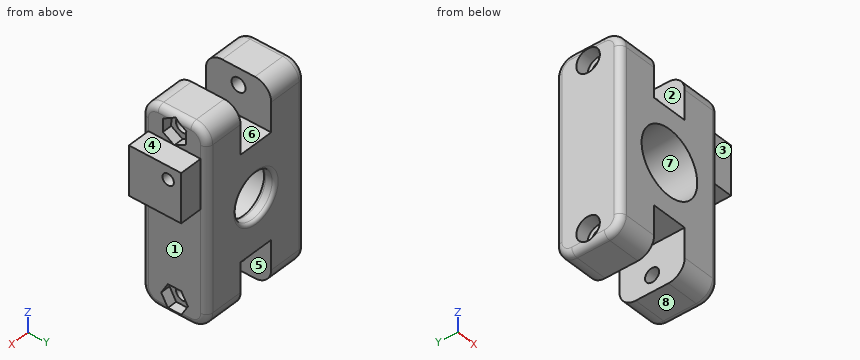
from build123d import *

# Parameters (mm, degrees)
SKETCH1_W           = 35
SKETCH1_H           = 60
BOSS_EXTRUDE1_DEPTH = 20
SKETCH2_R           = 10
CUT_EXTRUDE1_DEPTH  = 16
SKETCH4_R           = 7
CUT_EXTRUDE2_DEPTH  = 42.997755111
FILLET1_R           = 2
SKETCH5_W           = 11
SKETCH5_H           = 14
CUT_EXTRUDE3_DEPTH  = 44.678500826
SKETCH6_R           = 2.15
CUT_EXTRUDE4_DEPTH  = 53.234749007
FILLET3_R           = 5
FILLET4_R           = 5
FILLET7_R           = 1
SKETCH9_W           = 15
SKETCH9_H           = 16
BOSS_EXTRUDE3_DEPTH = 7
SKETCH10_R          = 1.75
CUT_EXTRUDE6_DEPTH  = 5
SKETCH12_R          = 3.6
CUT_EXTRUDE7_DEPTH  = 4
CUT_EXTRUDE8_DEPTH  = 3


with BuildPart() as part:
    # Sketch1 → Boss-Extrude1 (new body)
    with BuildSketch(Plane(origin=(0, 0, 0), x_dir=(1, 0, 0), z_dir=(0, 1, 0))):
        with Locations((-2.608267717, 3.218503937)):
            Rectangle(SKETCH1_W, SKETCH1_H)
    extrude(amount=BOSS_EXTRUDE1_DEPTH)

    # Sketch2 → Cut-Extrude1 (cut)
    with BuildSketch(Plane.XZ):
        with Locations(Location((-2.608267717, -3.218503937, 0), (0, 0, 270))):
            Circle(SKETCH2_R)
    extrude(amount=-CUT_EXTRUDE1_DEPTH, mode=Mode.SUBTRACT)

    # Sketch4 → Cut-Extrude2 (cut, through all)
    with BuildSketch(Plane.XZ.offset(-16)):
        with Locations(Location((-2.608267717, -3.218503937, 0), (0, 0, 270))):
            Circle(SKETCH4_R)
    extrude(amount=-CUT_EXTRUDE2_DEPTH, mode=Mode.SUBTRACT)

    # Fillet1
    fillet1_edges = [part.edges().sort_by_distance(p)[0] for p in [
        (-20.108267717, 20, -3.218503937),
        (14.891732283, 20, -3.218503937),
        (-20.108267717, 0, -3.218503937),
        (14.891732283, 0, -3.218503937),
        (14.891732283, 10, 26.781496063),
        (-20.108267717, 10, 26.781496063),
        (-20.108267717, 10, -33.218503937),
        (14.891732283, 10, -33.218503937),
    ]]
    fillet(fillet1_edges, radius=FILLET1_R)

    # Sketch5 → Cut-Extrude3 (cut, through all)
    with BuildSketch(Plane.XZ):
        with Locations((-2.608267717, 19.781496063)):
            Rectangle(SKETCH5_W, SKETCH5_H)
        with Locations((-2.608267717, -26.218503937)):
            Rectangle(SKETCH5_W, SKETCH5_H)
    extrude(amount=-CUT_EXTRUDE3_DEPTH, mode=Mode.SUBTRACT)

    # Sketch6 → Cut-Extrude4 (cut, through all)
    with BuildSketch(Plane.ZY.offset(20.108267717)):
        with Locations((-28.218503937, 10)):
            Circle(SKETCH6_R)
        with Locations((21.781496063, 10)):
            Circle(SKETCH6_R)
    extrude(amount=-CUT_EXTRUDE4_DEPTH, mode=Mode.SUBTRACT)

    # Fillet3
    # the kernel refuses this fillet: 5 mm, written as the material it takes off along each edge
    with BuildSketch(Plane(origin=(-20.108267717, 15, 21.781496063), x_dir=(0, 0, 1), z_dir=(0, -1, 0))) as fillet3_piece_1:
        with BuildLine():
            CenterArc((3, -2), 2, 0, 90)
            Line((5, -2), (5, 0))
            Line((5, 0), (3, 0))
        make_face()
    revolve(axis=Axis((-20.108267717, 15, 21.781496063), (-1, 0, 0)), revolution_arc=90, mode=Mode.SUBTRACT)
    with BuildSketch(Plane(origin=(-20.108267717, 5, 21.781496063), x_dir=(0, -1, 0), z_dir=(0, 0, -1))) as fillet3_piece_2:
        with BuildLine():
            CenterArc((3, -2), 2, 0, 90)
            Line((5, -2), (5, 0))
            Line((5, 0), (3, 0))
        make_face()
    revolve(axis=Axis((-20.108267717, 5, 21.781496063), (-1, 0, 0)), revolution_arc=90, mode=Mode.SUBTRACT)
    with BuildSketch(Plane(origin=(14.891732283, 15, 21.781496063), x_dir=(0, 1, 0), z_dir=(0, 0, -1))) as fillet3_piece_3:
        with BuildLine():
            CenterArc((3, -2), 2, 0, 90)
            Line((5, -2), (5, 0))
            Line((5, 0), (3, 0))
        make_face()
    revolve(axis=Axis((14.891732283, 15, 21.781496063), (1, 0, 0)), revolution_arc=90, mode=Mode.SUBTRACT)
    with BuildSketch(Plane(origin=(14.891732283, 5, 21.781496063), x_dir=(0, 0, 1), z_dir=(0, 1, 0))) as fillet3_piece_4:
        with BuildLine():
            CenterArc((3, -2), 2, 0, 90)
            Line((5, -2), (5, 0))
            Line((5, 0), (3, 0))
        make_face()
    revolve(axis=Axis((14.891732283, 5, 21.781496063), (1, 0, 0)), revolution_arc=90, mode=Mode.SUBTRACT)
    with BuildSketch(Plane(origin=(4.391732283, 20, 26.781496063), x_dir=(0, 0, -1), z_dir=(-1, 0, 0)), Plane(origin=(14.891732283, 0, 26.781496063), x_dir=(0, 1, 0), z_dir=(-1, 0, 0))) as fillet3_piece_5:
        with BuildLine():
            CenterArc((FILLET3_R, FILLET3_R), FILLET3_R, 180, 90)
            Line((0, FILLET3_R), (0, 0))
            Line((0, 0), (FILLET3_R, 0))
        make_face()
    extrude(amount=24.5, mode=Mode.SUBTRACT)
    with BuildSketch(Plane(origin=(4.391732283, 0, 26.781496063), x_dir=(0, 0, -1), z_dir=(-1, 0, 0)), Plane(origin=(14.891732283, 20, 26.781496063), x_dir=(0, -1, 0), z_dir=(-1, 0, 0))) as fillet3_piece_6:
        with BuildLine():
            CenterArc((FILLET3_R, -FILLET3_R), FILLET3_R, 90, 90)
            Line((0, -FILLET3_R), (0, 0))
            Line((0, 0), (FILLET3_R, 0))
        make_face()
    extrude(amount=24.5, mode=Mode.SUBTRACT)

    # Fillet4
    # the kernel refuses this fillet: 5 mm, written as the material it takes off along each edge
    with BuildSketch(Plane(origin=(-20.108267717, 15, -28.218503937), x_dir=(0, 1, 0), z_dir=(0, 0, 1))) as fillet4_piece_1:
        with BuildLine():
            CenterArc((3, -2), 2, 0, 90)
            Line((5, -2), (5, 0))
            Line((5, 0), (3, 0))
        make_face()
    revolve(axis=Axis((-20.108267717, 15, -28.218503937), (-1, 0, 0)), revolution_arc=90, mode=Mode.SUBTRACT)
    with BuildSketch(Plane(origin=(-20.108267717, 5, -28.218503937), x_dir=(0, 0, -1), z_dir=(0, 1, 0))) as fillet4_piece_2:
        with BuildLine():
            CenterArc((3, -2), 2, 0, 90)
            Line((5, -2), (5, 0))
            Line((5, 0), (3, 0))
        make_face()
    revolve(axis=Axis((-20.108267717, 5, -28.218503937), (-1, 0, 0)), revolution_arc=90, mode=Mode.SUBTRACT)
    with BuildSketch(Plane(origin=(14.891732283, 15, -28.218503937), x_dir=(0, 0, -1), z_dir=(0, -1, 0))) as fillet4_piece_3:
        with BuildLine():
            CenterArc((3, -2), 2, 0, 90)
            Line((5, -2), (5, 0))
            Line((5, 0), (3, 0))
        make_face()
    revolve(axis=Axis((14.891732283, 15, -28.218503937), (1, 0, 0)), revolution_arc=90, mode=Mode.SUBTRACT)
    with BuildSketch(Plane(origin=(14.891732283, 5, -28.218503937), x_dir=(0, -1, 0), z_dir=(0, 0, 1))) as fillet4_piece_4:
        with BuildLine():
            CenterArc((3, -2), 2, 0, 90)
            Line((5, -2), (5, 0))
            Line((5, 0), (3, 0))
        make_face()
    revolve(axis=Axis((14.891732283, 5, -28.218503937), (1, 0, 0)), revolution_arc=90, mode=Mode.SUBTRACT)
    with BuildSketch(Plane(origin=(-9.608267717, 0, -33.218503937), x_dir=(0, 1, 0), z_dir=(1, 0, 0)), Plane(origin=(-20.108267717, 0, -33.218503937), x_dir=(0, 1, 0), z_dir=(1, 0, 0))) as fillet4_piece_5:
        with BuildLine():
            CenterArc((FILLET4_R, FILLET4_R), FILLET4_R, 180, 90)
            Line((0, FILLET4_R), (0, 0))
            Line((0, 0), (FILLET4_R, 0))
        make_face()
    extrude(amount=24.5, mode=Mode.SUBTRACT)
    with BuildSketch(Plane(origin=(-9.608267717, 20, -33.218503937), x_dir=(0, -1, 0), z_dir=(1, 0, 0)), Plane(origin=(-20.108267717, 20, -33.218503937), x_dir=(0, -1, 0), z_dir=(1, 0, 0))) as fillet4_piece_6:
        with BuildLine():
            CenterArc((FILLET4_R, -FILLET4_R), FILLET4_R, 90, 90)
            Line((0, -FILLET4_R), (0, 0))
            Line((0, 0), (FILLET4_R, 0))
        make_face()
    extrude(amount=24.5, mode=Mode.SUBTRACT)

    # Fillet7
    fillet7_edges = [part.edges().sort_by_distance(p)[0] for p in [
        (-2.608267717, 20, 3.781496063),
        (-2.608267717, 16, 3.781496063),
    ]]
    fillet(fillet7_edges, radius=FILLET7_R)

    # Sketch9 → Boss-Extrude3 (add)
    with BuildSketch(Plane(origin=(14.891732283, 0, 0), x_dir=(0, 0, -1), z_dir=(1, 0, 0))):
        with Locations((-10.281496063, 10)):
            Rectangle(SKETCH9_W, SKETCH9_H)
    extrude(amount=BOSS_EXTRUDE3_DEPTH)

    # Sketch10 → Cut-Extrude6 (cut)
    with BuildSketch(Plane(origin=(21.891732283, 0, 0), x_dir=(0, 0, -1), z_dir=(1, 0, 0))):
        with Locations((-13.781496063, 14)):
            Circle(SKETCH10_R)
    extrude(amount=-CUT_EXTRUDE6_DEPTH, mode=Mode.SUBTRACT)

    # Sketch12 → Cut-Extrude7 (cut)
    with BuildSketch(Plane.ZY.offset(20.108267717)):
        with Locations((-28.218503937, 10)):
            Circle(SKETCH12_R)
        with Locations((21.781496063, 10)):
            Circle(SKETCH12_R)
    extrude(amount=-CUT_EXTRUDE7_DEPTH, mode=Mode.SUBTRACT)

    # Sketch13 → Cut-Extrude8 (cut)
    with BuildSketch(Plane(origin=(14.891732283, 0, 0), x_dir=(0, 0, -1), z_dir=(1, 0, 0))):
        Polygon((-19.793991712, 6.414869628), (-17.682929909, 9.928664072), (-19.67043426, 13.513794445), (-23.769000414, 13.585130372), (-25.880062217, 10.071335928), (-23.892557866, 6.486205555), align=None)
        Polygon((28.218503937, 5.900813089), (31.768503937, 7.950406544), (31.768503937, 12.049593456), (28.218503937, 14.099186911), (24.668503937, 12.049593456), (24.668503937, 7.950406544), align=None)
    extrude(amount=-CUT_EXTRUDE8_DEPTH, mode=Mode.SUBTRACT)


solid = part.part
Input: part model. Units: mm. Frame: model coordinates. Face numbers are marked on the shaded views. A direction names the side the tool comes from. Coordinates: 2 decimals unless noted, no trailing zeros. Loops run counter-clockwise (first coordinate to the right, second up) from the corner with the lowest first, then second, coordinate; pieces in that order, holes last. Notation, with made-up numbers: (-25.75, 0) -> (-0.75, 0) arc R7 ccw to (-0.75, 6) -> close; hole circle Ø3 at (66.5, -28.5). An arc over 180 degrees is marked (long way). One line per item, written item: value.
(1) Set-up query: the marked faces 1, 2, 3, 4 and 5. Return all of +Z, -Z, +X, -X, +Y, -Y with unobstructed straight access to the full face (end or side cutting, diameter ignored); none if empty.
Answer below:
face 1: -Z, +X, +Y, -Y
face 2: +Z, +Y, -Y
face 3: +Z, -Z, +X, -Y
face 4: +Z, +X, +Y, -Y
face 5: -Z, +Y, -Y
(2) Cut plane C-C (z = 10.5). Output: boundary loops of the cut face in (x, y), then the cut area to 3 significant figures.
Answer below:
outline: (-20.11, 2) arc R2 ccw to (-18.11, 0) -> (12.89, 0) arc R2 ccw to (14.89, 2) -> (21.89, 2) -> (21.89, 18) -> (14.89, 18) arc R2 ccw to (12.89, 20) -> (-18.11, 20) arc R2 ccw to (-20.11, 18) -> close
area: 809 mm2
(3) Draft query along Z for the marked faces 6, 7 and 8. Return one class per face: pulls with the +Z half, pulls with the -Z half, needs draft (parallel to the pull), parting line crosses it, or undercut.
Answer below:
face 6: pulls with the +Z half
face 7: undercut
face 8: pulls with the -Z half
(4) Ray query, line 1 along X through (y, z) = (14.5, -30); line 2 along X through (y, z) = (7.5, -15.5); line 3 along X through (y, z) = (8, -4). Return the intervals inside material, ascending.
Answer below:
line 1: x = -20.11 to -8.11, 2.89 to 14.89
line 2: x = -20.11 to 14.89
line 3: x = -20.11 to -12.58, 7.36 to 14.89
(5) Pin query (flat end, axial travel): pin 1 Ø1 at (x, y) = (15, 6.5) entering from -Z; pin 2 Ø6.5 at (y, z) = (10, 21.78) entering from -X; pin 3 Ø5.5 at (y, z) = (10, 21.78) entering from +X. Return the tip coordinate at first contact, or that it passes through.
Answer below:
pin 1: stops at z = -32.41
pin 2: stops at x = -16.11
pin 3: stops at x = 11.89
(6) Cut plane A-A (z = -15). Output: boundary loops of the cut face in (x, y).
Answer below:
outline: (-20.11, 2) arc R2 ccw to (-18.11, 0) -> (12.89, 0) arc R2 ccw to (14.89, 2) -> (14.89, 18) arc R2 ccw to (12.89, 20) -> (-18.11, 20) arc R2 ccw to (-20.11, 18) -> close
(7) Cut plane B-B (x = 19). Output: boundary loops of the cut face in (y, z), then the cut area to 3 significant figures.
Answer below:
outline: (2, 2.78) -> (18, 2.78) -> (18, 17.78) -> (2, 17.78) -> close; hole circle Ø3.5 at (14, 13.78)
area: 230 mm2
